Check sheet for the modelled part. Datum: model origin and axes. Units: mm. Face numbers are marked on the shaded views. A direction names the side the tool comes from. Give positions to 0.01 mm unless a question says otherwise; leave off trailing zeros. Write each loop counter-clockwise with the first axis right and the second up, starting at its lowest first coordinate (ties: lowest second). Pieces come first, ordered by that corner, then holes. Notation, with made-up numbers: (-26.75, 10) -> (25.25, 10) arc R22 ccw to (25.25, 39) -> close; hole circle Ø3 at (49.5, 2). An arc over 180 degrees is marked (long way). Use a Markdown table: item, result. Add a question column.
1. Cross-section at B-B (y = 20.5). Enter the section's corners in (x, z).
2. Cross-section at C-C (z = 4.5). Enter the section's corners in (x, y).
3. Cross-section at A-A (x = 76.5). Enter the section's corners in (y, z), then the cut area to 3 significant figures.
4. Set-up check for the marked faces 1 and 2: record each of +Z, -Z, +X, -X, +Y, -Y from which the full face is reachable in a straight line by a thin tool's end or side.
5. Gauge pin test, flat ends, axial feed: P1, Ø5, axis at x = 76, y = 21, coming from the -Z side; P2, Ø3, axis at y = 7, z = 1, coming from the +X side; P3, Ø3, axis at x = 35, z = 1.5, coming from the +Y side. Record the tip position at first contact, or that the pin passes through.
6. Scan lines: probe 1 along X at (y, z) = (13, 1.5); probe 2 along Z at (x, y) = (46.5, 18.5); probe 3 along X at (y, z) = (18, 4.5). Record each from-to range of solid material in increasing order. Write a range as [from, to].
from build123d import *

# Parameters (mm, degrees)
BOSS_EXTRUDE1_DEPTH = 144.78
SKETCH2_W           = 30.48
SKETCH2_H           = 11.43
BOSS_EXTRUDE2_DEPTH = 2.54


with BuildPart() as part:
    # Sketch1 → Boss-Extrude1 (new body)
    with BuildSketch(Plane.YZ):
        Polygon((0, 0), (17.78, 0), (17.78, 7.62), (24.13, 7.62), (24.13, 13.97), (17.78, 13.97), (0, 13.97), (-6.35, 13.97), (-6.35, 7.62), (0, 7.62), align=None)
    extrude(amount=BOSS_EXTRUDE1_DEPTH)

    # Sketch2 → Boss-Extrude2 (add)
    with BuildSketch(Plane.YZ.offset(144.78)):
        with Locations((8.89, 8.255)):
            Rectangle(SKETCH2_W, SKETCH2_H)
    extrude(amount=BOSS_EXTRUDE2_DEPTH)


solid = part.part
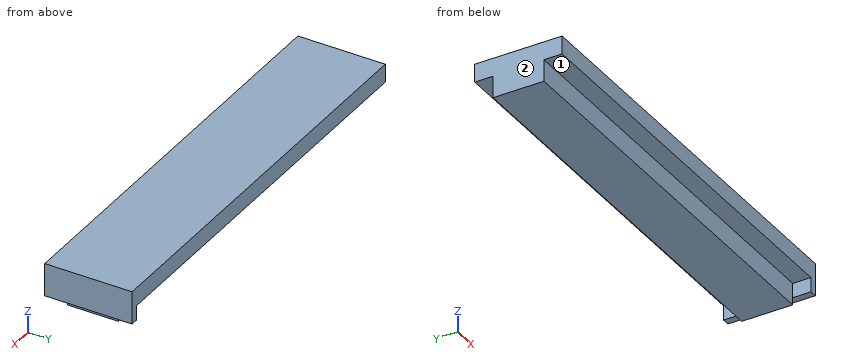
Worked answers:
| question | item | result |
|---|---|---|
| 1 | outline | (0, 7.62) -> (144.78, 7.62) -> (144.78, 2.54) -> (147.32, 2.54) -> (147.32, 13.97) -> (0, 13.97) -> close |
| 2 | outline | (0, 0) -> (144.78, 0) -> (144.78, -6.35) -> (147.32, -6.35) -> (147.32, 24.13) -> (144.78, 24.13) -> (144.78, 17.78) -> (0, 17.78) -> close |
| 3 | outline | (-6.35, 7.62) -> (0, 7.62) -> (0, 0) -> (17.78, 0) -> (17.78, 7.62) -> (24.13, 7.62) -> (24.13, 13.97) -> (-6.35, 13.97) -> close |
| 3 | area | 329 mm² |
| 4 | face 1 | -Z, -X, -Y |
| 4 | face 2 | +Z, -Z, -X, +Y, -Y |
| 5 | P1 | stops at z = 7.62 |
| 5 | P2 | stops at x = 144.78 |
| 5 | P3 | stops at y = 17.78 |
| 6 | probe 1 | x = [0, 144.78] |
| 6 | probe 2 | z = [7.62, 13.97] |
| 6 | probe 3 | x = [144.78, 147.32] |
